Source: CAD feature listing. Evaluate the final solid. Frame: model axes, mm. A direction names the side the tool comes from. Give positions to 0.01 mm unless a question says otherwise; leave off trailing zeros. Order: outer loops, then holes, each group sorted by start corner. A loop starts at its lowest first (then second) coordinate and runs counter-clockwise, first axis right, second up. Notation, with made-up numbers: (2.5, 73.25) -> (21.5, 73.25) arc R29 ccw to (21.5, 101.25) -> close; hole circle Ø6 at (88.25, 5). An arc over 180 degrees is marked (long way). Answer in a Markdown table with one row per item.
```python
from build123d import *

# Parameters (mm, degrees)
F0_W    = 15.4116954654
F0_H    = 29.5077543706
F0_W_2  = 59.3914035708
F0_H_2  = 28.9439186454
F2_SIZE = 5


with BuildPart() as f1:
    # F0 (on Right) → F1 (revolve)
    with BuildSketch(Plane.YZ):
        with Locations((7.7058477327, 30.91736231)):
            Rectangle(F0_W, F0_H)
        with Locations((45.1073972508, 30.91736231)):
            Rectangle(F0_W_2, F0_H)
        with Locations((7.7058477327, 60.143198818)):
            Rectangle(F0_W, F0_H_2)
    revolve(axis=Axis((0, 37.4015495181, 0), (0, 1, 0)))

    # F2
    f2_edges = [f1.edges().sort_by_distance(p)[0] for p in [
        (0, 15.411695, -45.671239),
        (0, 74.803099, -45.671239),
    ]]
    chamfer(f2_edges, length=F2_SIZE)


solid = f1.part
```
(1) Section query C-C (y = 45). Return the cut outline in (x, z), plus the area to 3 significant figures.
A:
| item | result |
|---|---|
| outline | circle Ø91.34 at (0, 0); hole circle Ø32.33 at (0, 0) |
| area | 5,730 mm^2 |
(2) Section query A-A (z = 0). Return the cut outline in (x, y).
A:
| item | result |
|---|---|
| outline | (-74.62, 0) -> (-16.16, 0) -> (-16.16, 74.8) -> (-40.67, 74.8) -> (-45.67, 69.8) -> (-45.67, 20.41) -> (-50.67, 15.41) -> (-74.62, 15.41) -> close; (16.16, 0) -> (74.62, 0) -> (74.62, 15.41) -> (50.67, 15.41) -> (45.67, 20.41) -> (45.67, 69.8) -> (40.67, 74.8) -> (16.16, 74.8) -> close |
(3) Access query for faces 1 (the flat face through (-16, 15.412, -49)), 2 (the flat face through (-18, 74.803, 1)). Directions: +Z, -Z, +X, -X, +Y, -Y. A direction counts if a zero-diameter tool reaches every point of the face in a straight line with its end or side. Return the directions, or none.
A:
| item | result |
|---|---|
| face 1 | +Y |
| face 2 | +Z, -Z, +X, -X, +Y |
(4) Section query B-B (x = 0). Return the cut outline in (y, z), plus the area to 3 significant figures.
A:
| item | result |
|---|---|
| outline | (0, -74.62) -> (15.41, -74.62) -> (15.41, -50.67) -> (20.41, -45.67) -> (69.8, -45.67) -> (74.8, -40.67) -> (74.8, -16.16) -> (0, -16.16) -> close; (0, 16.16) -> (74.8, 16.16) -> (74.8, 40.67) -> (69.8, 45.67) -> (20.41, 45.67) -> (15.41, 50.67) -> (15.41, 74.62) -> (0, 74.62) -> close |
| area | 5,310 mm^2 |
(5) First-contact query: pin 1 Ø12 at (x, z) = (16.5, -33) entering from -Y; pin 2 Ø4 at (y, z) = (42, 11) entering from +X; pin 3 Ø3 at (y, z) = (32.5, 34.5) entering from +X; pin 4 Ø5 at (y, z) = (58.5, -16) entering from -X. Flat tips, straight axial feed; report the tip coordinate or a pass-through.
A:
| item | result |
|---|---|
| pin 1 | stops at y = 0 |
| pin 2 | stops at x = 44.78 |
| pin 3 | stops at x = 31.57 |
| pin 4 | stops at x = -43.63 |
(6) Section query D-D (z = -57). Return the cut outline in (x, y), plus the area to 3 significant figures.
A:
| item | result |
|---|---|
| outline | (-48.15, 0) -> (48.15, 0) -> (48.15, 15.41) -> (-48.15, 15.41) -> close |
| area | 1,480 mm^2 |
(7) Ray query, probe 1 along X at (y, z) = (15, 0); probe 2 along X at (y, z) = (25.5, 0); probe 3 along Y at (x, z) = (-22, -59.5). Return the intervals inside material, ascending.
A:
| item | result |
|---|---|
| probe 1 | x = -74.62 to -16.16, 16.16 to 74.62 |
| probe 2 | x = -45.67 to -16.16, 16.16 to 45.67 |
| probe 3 | y = 0 to 15.41 |
(8) Pull-direction query (X, two-part tool) for faces 3 (the flat face through (18, 0, -1)), 4 (the conical face through (-36.36, 74.49, 18.91)), 5 (the cylindrical face through (16.026, 37.925, -2.104)); classes: +X half, -X half, draft (parallel to the pull), parting line (faces both ways), or undercut.
A:
| item | result |
|---|---|
| face 3 | draft |
| face 4 | parting line |
| face 5 | undercut |
